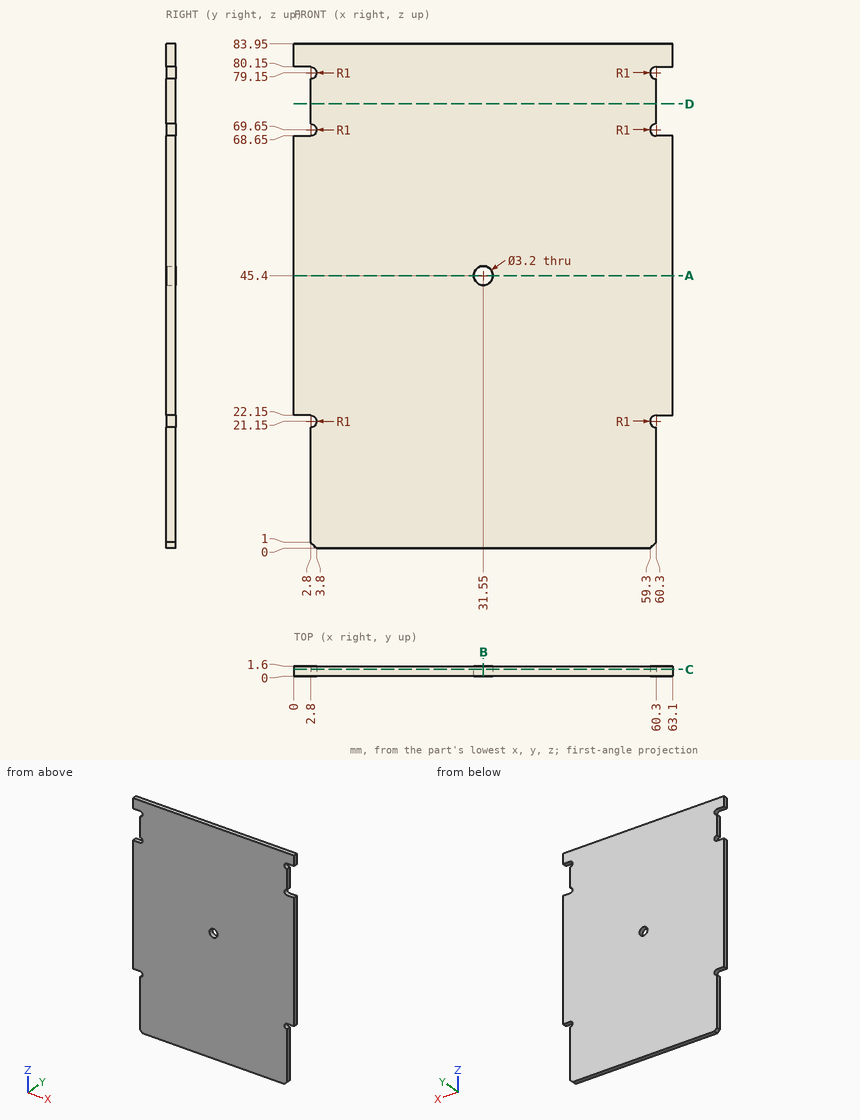
Verification items for this drawing (mm, ordinates from the low corner). Coordinates: 2 decimals unless noted, no trailing zeros. Write each loop counter-clockwise with the first axis right and the second up, starting at its lowest first coordinate (ties: lowest second). Pieces come first, ordered by that corner, then holes. Notation, with made-up numbers: M 15,-29.5 L 59,-29.5 A17 cw 59,0.5 Z; hole C 80,-14.5 d11. An arc over 180 degrees is marked long. Answer as a JSON object with one key per item and string values.
1. Section check C-C, the plane y = 1.1. Enter the section's corners in (x, z), plus the area to 3 significant figures.
Answers below:
{"outline": "M 0,22.15 L 2.8,22.15 A1 cw 2.8,20.15 L 2.8,1 L 3.8,0 L 59.3,0 L 60.3,1 L 60.3,20.15 A1 cw 60.3,22.15 L 63.1,22.15 L 63.1,68.65 L 60.3,68.65 A1 cw 60.3,70.65 L 60.3,78.15 A1 cw 60.3,80.15 L 63.1,80.15 L 63.1,83.95 L 0,83.95 L 0,80.15 L 2.8,80.15 A1 cw 2.8,78.15 L 2.8,70.65 A1 cw 2.8,68.65 L 0,68.65 Z; hole C 31.55,45.4 d3.2", "area": "5,090 mm²"}
2. Scan lines: L1, parallel to Z at x = 31.55, y = 0.75; L2, parallel to Z at x = 60, y = 1.15; L3, parallel to X at y = 0.5, z = 4. Record each from-to range of solid material in increasing order.
Answers below:
{"L1": "z = 0 to 43.8, 47 to 83.95", "L2": "z = 0.7 to 20.2, 22.1 to 68.7, 70.6 to 78.2, 80.1 to 83.95", "L3": "x = 2.8 to 60.3"}
3. Section check B-B, the plane x = 31.55. Enter the section's corners in (y, z), plus the area to 3 significant figures.
Answers below:
{"outline": "M 0,0 L 1.6,0 L 1.6,43.8 L 0,43.8 Z; M 0,47 L 1.6,47 L 1.6,83.95 L 0,83.95 Z", "area": "129 mm²"}
4. Section check A-A, the plane z = 45.4. Enter the section's corners in (x, y).
Answers below:
{"outline": "M 0,0 L 29.95,0 L 29.95,1.6 L 0,1.6 Z; M 33.15,0 L 63.1,0 L 63.1,1.6 L 33.15,1.6 Z"}
5. Go/stop test with flat-tipped pins: pin 1 Ø0.5 at (y, z) = (1, 12.5) entering from +X; pin 2 Ø0.8 at (y, z) = (0.5, 75.5) entering from -X; pin 3 Ø0.5 at (x, y) = (61.5, 1) entering from -Z. Record where each tip stops, or that it passes through.
Answers below:
{"pin 1": "stops at x = 60.3", "pin 2": "stops at x = 2.8", "pin 3": "stops at z = 22.15"}
6. Section check D-D, the plane z = 74. Enter the section's corners in (x, y), plus the area to 3 significant figures.
Answers below:
{"outline": "M 2.8,0 L 60.3,0 L 60.3,1.6 L 2.8,1.6 Z", "area": "92.0 mm²"}
